Work out the finished part from the listing and answer in its coordinate system (mm). Face numbers are marked on the shaded views. A direction names the side the tool comes from. Coordinates: 2 decimals unless noted, no trailing zeros. Order: outer loops, then holes, each group sorted by start corner. A loop starts at its lowest first (then second) coordinate and runs counter-clockwise, first axis right, second up. Notation, with made-up numbers: M 27,-38 L 68,-38 A5 cw 68,-33 Z; hole C -10,-27.5 d3. An arc over 180 degrees is marked long. Write item = value, one per line. Start each with the question number.
Q1. Each of these flat-tipped pins is pushed along its axis until it touches: P1, Ø3, axis at x = 56, y = -20, coming from the +Z side; P2, Ø6, axis at y = 79.5, z = 10, coming from the -X side; P3, Ø10, axis at x = 38.5, z = 26.5, coming from the -Y side. Where does it stop, or does it pass through?
Q2. A tool of negligible diameter and unlimited length cuts with its end or side. For the marked faces 1, 2 and 3, from which of +Z, -Z, +X, -X, +Y, -Y can it reach the whole face along a straight path? Write none if from no direction.
Q3. Find section C-C on z = 17. Give the vertices of the cut face in (x, y), and give its area (3 significant figures).
Q4. Find section B-B on y = -75. Give the vertices of the cut face in (x, z).
Q5. Find section D-D on y = 6.5. Give the vertices of the cut face in (x, z), and give its area (3 significant figures).
Q6. Determine the mould class of the marked faces 4, 5 and 6 for opening direction Y: released by +Y, released by -Y, zero draft, split by the parting line, or undercut.
Q7. Straight lines are drawn through the part: line 1 along Y through (x, z) = (78.75, 1); line 2 along Y through (x, z) = (-78.75, 0.8); line 3 along Z through (x, y) = (-7.5, 18.5). For each, find the intervals that lie inside material, in ascending order.
Q8. Find section A-A on x = -78.75. Give the vertices of the cut face in (y, z), and give its area (3 significant figures).
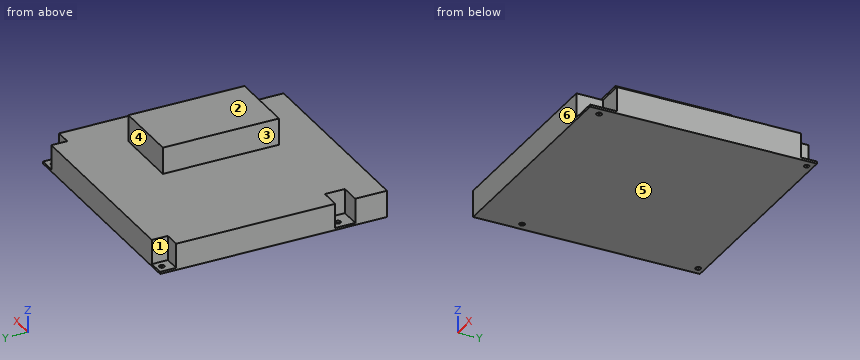
```python
from build123d import *

# Parameters (mm, degrees)
SKETCH_1_W          = 170
SKETCH_1_H          = 170
EXTRUDE_1_DEPTH     = 20
SKETCH_2_W          = 20
SKETCH_2_H          = 20
SKETCH_2_W_2        = 12
SKETCH_2_H_2        = 12
SKETCH_2_W_3        = 15
SKETCH_2_H_3        = 15
CUT_EXTRUDE_1_DEPTH = 18.4
SKETCH_3_R          = 2
SKETCH_3_R_2        = 1.82271494
CUT_EXTRUDE_2_DEPTH = 18.4
SKETCH_4_W          = 50
SKETCH_4_H          = 87
EXTRUDE_2_DEPTH     = 20


with BuildPart() as part:
    # 草圖1 → 填料-伸長1 (new body)
    with BuildSketch(Plane.XY):
        Rectangle(SKETCH_1_W, SKETCH_1_H)
    extrude(amount=EXTRUDE_1_DEPTH)

    # 草圖2 → 除料-伸長1 (cut)
    with BuildSketch(Plane.XY.offset(20)):
        with Locations((75, -75)):
            Rectangle(SKETCH_2_W, SKETCH_2_H)
        with Locations((79, 79)):
            Rectangle(SKETCH_2_W_2, SKETCH_2_H_2)
        with Locations((-79, 79)):
            Rectangle(SKETCH_2_W_2, SKETCH_2_H_2)
        with Locations((-77.5, -53.711717692)):
            Rectangle(SKETCH_2_W_3, SKETCH_2_H_3)
    extrude(amount=-CUT_EXTRUDE_1_DEPTH, mode=Mode.SUBTRACT)

    # 草圖3 → 除料-伸長2 (cut)
    with BuildSketch(Plane.XY.offset(1.6)):
        with Locations((78.75, -75)):
            Circle(SKETCH_3_R)
        with Locations((78.75, 80.5)):
            Circle(SKETCH_3_R_2)
        with Locations((-78.75, 80.5)):
            Circle(SKETCH_3_R)
        with Locations((-78.75, -51.5)):
            Circle(SKETCH_3_R)
    extrude(amount=-CUT_EXTRUDE_2_DEPTH, mode=Mode.SUBTRACT)

    # 草圖4 → 填料-伸長2 (add)
    with BuildSketch(Plane.XY.offset(20)):
        with Locations((29, -6.5)):
            Rectangle(SKETCH_4_W, SKETCH_4_H)
    extrude(amount=EXTRUDE_2_DEPTH)


solid = part.part
```
Findings below:
q1.P1 = 20
q1.P2 = -73
q1.P3 = -50
q2.face_1 = +Z, -X, +Y
q2.face_2 = +Z, +X, -X, +Y, -Y
q2.face_3 = +Z, -X, +Y, -Y
q3.outline = M -85,-85 L 65,-85 L 65,-65 L 85,-65 L 85,73 L 73,73 L 73,85 L -73,85 L -73,73 L -85,73 L -85,-46.21 L -70,-46.21 L -70,-61.21 L -85,-61.21 Z
q3.area = 28,000 mm^2
q4.outline = M -85,0 L 76.75,0 L 76.75,1.6 L 65,1.6 L 65,20 L -85,20 Z; M 80.75,0 L 85,0 L 85,1.6 L 80.75,1.6 Z
q5.outline = M -85,0 L 85,0 L 85,20 L 54,20 L 54,40 L 4,40 L 4,20 L -85,20 Z
q5.area = 4,400 mm^2
q6.face_4 = released by +Y
q6.face_5 = zero draft
q6.face_6 = released by -Y
q7.line_1 = -85 to -77, -73 to 78.68, 82.32 to 85
q7.line_2 = -85 to -53.5, -49.5 to 78.5, 82.5 to 85
q7.line_3 = 0 to 20
q8.outline = M -85,0 L -53.5,0 L -53.5,1.6 L -61.21,1.6 L -61.21,20 L -85,20 Z; M -49.5,0 L 78.5,0 L 78.5,1.6 L 73,1.6 L 73,20 L -46.21,20 L -46.21,1.6 L -49.5,1.6 Z; M 82.5,0 L 85,0 L 85,1.6 L 82.5,1.6 Z
q8.area = 2,890 mm^2
